Autodesk Inventor part; units mm, degrees
ref_plane "YZ Plane" through (0, 0, 0) normal (1, 0, 0) x (0, 1, 0)
ref_plane "XZ Plane" through (0, 0, 0) normal (0, 1, 0) x (-1, 0, 0)
ref_plane "XY Plane" through (0, 0, 0) normal (0, 0, 1) x (1, 0, 0)
sketch "Sketch1" plane through (0, 0, 0) normal (0, 0, 1) x (1, 0, 0)
  arc A0 (674.48, 374.6273) -> (275.278, 208.3151) centre (1116.653, -1248.9892) ccw
  line L0 (275.278, 208.3151) -> (0.0426, 49.4078)
  line L1 (0.0426, 49.4078) -> (28.6176, -0.0855)
  line L2 (28.6176, -0.0855) -> (303.853, 158.8217)
  arc A1 (695.9168, 321.2198) -> (303.853, 158.8217) centre (1116.653, -1248.9892) ccw
  line L3 (695.9168, 321.2198) -> (681.1253, 376.4225)
  arc A2 (681.1253, 376.4225) -> (275.278, 208.3151) centre (1116.653, -1248.9892) ccw
  line L4 (275.278, 208.3151) -> (0.0426, 49.4078)
  point P0 (0, 0)
extrude "Extrusion1" add sketch "Sketch1" along normal blind 19.05
properties part number "nd-15"
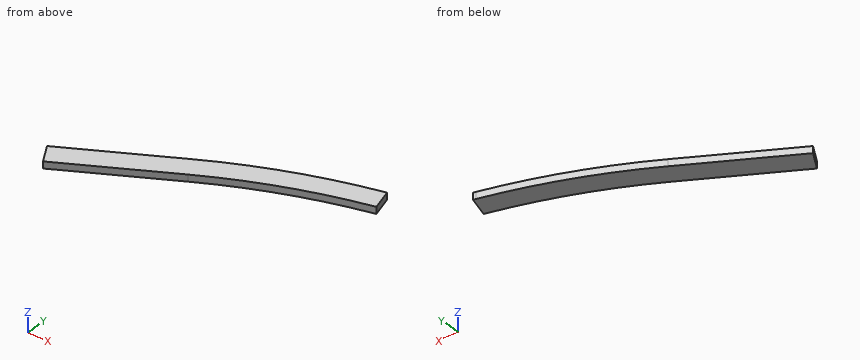
Geometry: final body of the model. Coordinates: model frame, mm. Give positions to 0.01 mm unless a question says otherwise; leave off trailing zeros. Order: outer loops, then holes, each group sorted by start corner. A loop starts at its lowest first (then second) coordinate and runs counter-clockwise, first axis right, second up. Notation, with made-up numbers: (-23, -14.75) -> (-17, -14.75) arc R20 cw to (-17, 10.25) -> close; hole circle Ø9 at (37, -22.75). An arc over 180 degrees is marked (long way). Write each question's results on one line, items separated by ' | '.
1) Cut plane A-A (z = 8.5). Output: boundary loops of the cut face in (x, y), and give its area (3 significant figures).
Geometry says:
outline: (0.04, 49.41) -> (28.62, -0.09) -> (303.85, 158.82) arc R1625.6 cw to (695.92, 321.22) -> (681.13, 376.42) arc R1682.75 ccw to (674.48, 374.63) arc R1682.75 ccw to (275.28, 208.32) -> close | area: 42,900 mm²
2) Cut plane C-C (x = 407.5). Output: boundary loops of the cut face in (y, z).
Geometry says:
outline: (213.77, 0) -> (277.03, 0) -> (277.03, 19.05) -> (213.77, 19.05) -> close
3) Line query: line 1 along X through (y, z) = (109, 15.75); line 2 along X through (y, z) = (97.5, 18.25); line 3 along Y through (x, z) = (481, 4). Output: solid intervals per line, ascending.
Geometry says:
line 1: x = 103.26 to 217.56 | line 2: x = 83.34 to 197.64 | line 3: y = 247.18 to 309.08
4) Cut plane B-B (y = 151). Output: boundary loops of the cut face in (x, z).
Geometry says:
outline: (176.01, 0) -> (290.31, 0) -> (290.31, 19.05) -> (176.01, 19.05) -> close
5) First-contact query: pin 1 Ø8 at (x, z) = (323.5, 16.5) entering from -Y; pin 2 Ø5 at (y, z) = (206.5, 4.5) entering from -X; pin 3 Ø8 at (x, z) = (624, 5) entering from +Y. Flat tips, straight axial feed; report the tip coordinate or a pass-through.
Geometry says:
pin 1: stops at y = 167.74 | pin 2: stops at x = 267.8 | pin 3: stops at y = 361.25
